Design review of the part built by this model. Coordinates are the model's own, in mm. A direction names the side the tool comes from. Coordinates: 2 decimals unless noted, no trailing zeros. Order: outer loops, then holes, each group sorted by start corner. A loop starts at its lowest first (then second) coordinate and runs counter-clockwise, first axis right, second up. Notation, with made-up numbers: (35, 4) -> (63, 4) arc R27 cw to (63, 32) -> close; hole circle Ø10 at (-0.75, 74). An arc over 180 degrees is marked (long way). Use a Markdown table: item, result. Add a question column.
Q1. Machinability: for faces 1 (the face through (-44.275, -1.503, -25.741)), 2 (the face through (-26.17, -1.5, 18.95)), which of the approach directions +Z, -Z, +X, -X, +Y, -Y give a long, thin tool a straight path to every point of the face, cutting with its end or side? Answer none if there is none.
Q2. Add section B-B (z = 35). State the section outline as (x, y) points, then the cut area to 3 significant figures.
Q3. Wall thickness on probe 1 along Z at (x, y) = (5, -2.65); probe 2 along Z at (x, y) = (-40, -2.4); probe 3 along Z at (x, y) = (-7, -0.7): over which ranges is each line inside the solid? List them lowest first.
Q4. Add section A-A (y = -1.1). Count the separate pieces of the cut face and the enclosed holes in it, then the cut area to 3 significant figures.
Q5. Insertion check: pin 1 (1 mm diameter, centred on x = -7.5, y = -2, fed in from +Z). The pin has a flat end and moves straight along its axis. Give the tip position at first contact, or say it passes through.
Q6. Add section C-C (x = -3). State the section outline as (y, z) points, then the cut area to 3 significant figures.
Q7. The part is to be moulded in two halves that separate along X. For faces 3 (the face through (-39.07, -1.5, 103.92)), 4 (the face through (-42.203, -1.503, -19.767)), 5 (the face through (-54.906, -1.503, 43.622)), say which applies: pulls with the +X half, pulls with the -X half, needs draft (parallel to the pull), parting line crosses it, or undercut.
from build123d import *

# Parameters (mm, degrees)
F0_R     = 3.175
F0_R_2   = 1.5875
F1_DEPTH = 3.048


with BuildPart() as f1:
    # F0 (on Front) → F1 (new body)
    with BuildSketch(Plane.XZ):
        with BuildLine():
            ThreePointArc((-48.556072, 94.40956), (-39.039076, 84.868582), (-29.506085, 94.393578))
            ThreePointArc((-29.506085, 94.393578), (-29.509424, 94.645752), (-29.519438, 94.897749))
            ThreePointArc((-29.519438, 94.897749), (-39.275271, 103.915448), (-48.556072, 94.40956))
        make_face()
        with Locations((-39.031085, 94.393578)):
            Circle(F0_R, mode=Mode.SUBTRACT)
        with BuildLine():
            ThreePointArc((-29.519438, 94.897749), (-29.509424, 94.645752), (-29.506085, 94.393578))
            ThreePointArc((-29.506085, 94.393578), (-39.039076, 84.868582), (-48.556072, 94.40956))
            Line((-48.556072, 94.40956), (-54.778624, 45.601225))
            ThreePointArc((-54.778624, 45.601225), (-39.023338, 59.468576), (-23.281594, 45.585853))
            Line((-23.281594, 45.585853), (-29.519438, 94.897749))
        make_face()
        with Locations((-45.03163, 80.118778)):
            Circle(F0_R_2, mode=Mode.SUBTRACT)
        with BuildLine():
            ThreePointArc((-23.156085, 43.593578), (-23.187494, 44.59169), (-23.281594, 45.585853))
            ThreePointArc((-23.281594, 45.585853), (-39.023338, 59.468576), (-54.778624, 45.601225))
            ThreePointArc((-54.778624, 45.601225), (-54.906085, 43.593578), (-54.778624, 41.585932))
            ThreePointArc((-54.778624, 41.585932), (-39.031085, 27.718578), (-23.283546, 41.585932))
            ThreePointArc((-23.283546, 41.585932), (-23.187983, 42.587734), (-23.156085, 43.593578))
        make_face()
        with Locations((-39.031085, 43.593578)):
            Circle(F0_R, mode=Mode.SUBTRACT)
        with BuildLine():
            ThreePointArc((-23.283546, 41.585932), (-39.031085, 27.718578), (-54.778624, 41.585932))
            Line((-54.778624, 41.585932), (-46.812516, -20.898473))
            ThreePointArc((-46.812516, -20.898473), (-39.52811, -12.077769), (-31.186671, -19.906422))
            ThreePointArc((-31.186671, -19.906422), (-33.484247, -25.45326), (-39.031085, -27.750836))
            Line((-39.031085, -27.750836), (5.402289, -27.843904))
            ThreePointArc((5.402289, -27.843904), (-2.518585, -19.906422), (5.402289, -11.968939))
            Line((5.402289, -11.968939), (-21.073536, -12.024395))
            ThreePointArc((-21.073536, -12.024395), (-27.051216, -9.334614), (-28.976555, -3.068783))
            Line((-28.976555, -3.068783), (-23.283546, 41.585932))
        make_face()
        with BuildLine():
            ThreePointArc((-31.186671, -19.906422), (-39.52811, -12.077769), (-46.812516, -20.898473))
            ThreePointArc((-46.812516, -20.898473), (-44.215329, -25.793564), (-39.031085, -27.750836))
            ThreePointArc((-39.031085, -27.750836), (-33.484247, -25.45326), (-31.186671, -19.906422))
        make_face()
        with Locations((-39.031085, -19.906422)):
            Circle(F0_R, mode=Mode.SUBTRACT)
        with BuildLine():
            ThreePointArc((5.402289, -11.968939), (-2.518585, -19.906422), (5.402289, -27.843904))
            ThreePointArc((5.402289, -27.843904), (11.025694, -25.524957), (13.356415, -19.906422))
            ThreePointArc((13.356415, -19.906422), (11.025694, -14.287887), (5.402289, -11.968939))
        make_face()
        with Locations((5.418915, -19.906422)):
            Circle(F0_R, mode=Mode.SUBTRACT)
    extrude(amount=F1_DEPTH)


solid = f1.part
Established:
| question | item | result |
|---|---|---|
| 1 | face 1 | -Z, -X, +Y, -Y |
| 1 | face 2 | +X, +Y, -Y |
| 2 | outline | (-53.94, -3.05) -> (-24.12, -3.05) -> (-24.12, 0) -> (-53.94, 0) -> close |
| 2 | area | 90.9 mm^2 |
| 3 | probe 1 | -27.84 to -23.05, -16.76 to -11.97 |
| 3 | probe 2 | -27.69 to -22.93, -16.88 to 40.57, 46.62 to 91.37, 97.42 to 103.87 |
| 3 | probe 3 | -27.82 to -11.99 |
| 4 | separate pieces | 1 |
| 4 | enclosed holes | 5 |
| 4 | area | 3,630 mm^2 |
| 5 | pin 1 | z = -11.99 |
| 6 | outline | (-3.05, -27.83) -> (0, -27.83) -> (0, -11.99) -> (-3.05, -11.99) -> close |
| 6 | area | 48.3 mm^2 |
| 7 | face 3 | parting line crosses it |
| 7 | face 4 | undercut |
| 7 | face 5 | pulls with the -X half |
